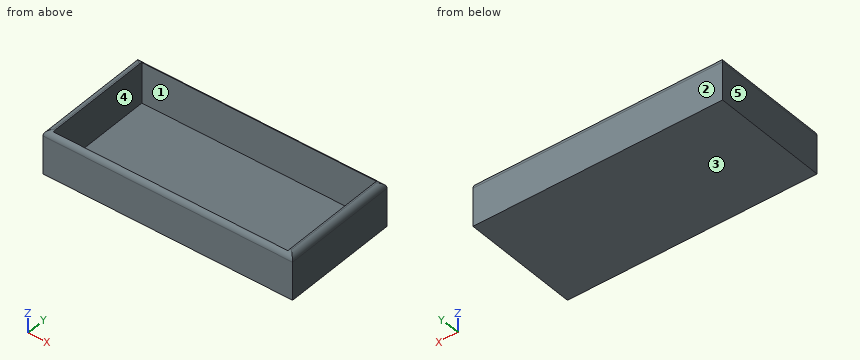
```python
from build123d import *

# Parameters (mm, degrees)
F0_W        = 170
F0_H        = 80
F1_DEPTH    = 30
F2_W        = 160
F2_H        = 75
F3_DEPTH    = 28
F4_T1_DEPTH = 190
F4_T3_DEPTH = 100


# Not quite as in the source:
# - a fillet or chamfer that OpenCascade refuses, or shapes differently, is made with other operations: its cross-section is extruded or revolved along the edge and cut away or added


with BuildPart() as f1:
    # F0 (on Top) → F1 (new body)
    with BuildSketch(Plane.XY):
        Rectangle(F0_W, F0_H)
    extrude(amount=F1_DEPTH)

    # F2 (on face) → F3 (cut)
    with BuildSketch(Plane.XY.offset(30)):
        Rectangle(F2_W, F2_H)
    extrude(amount=-F3_DEPTH, mode=Mode.SUBTRACT)

    # F4: fillet of radius 4 on 4 edges, made by hand

    # F4_s2 → F4_t1 (cut)
    with BuildSketch(Plane.YZ.offset(-95)):
        with BuildLine():
            ThreePointArc((-40, 26), (-38.8284271247, 28.8284271247), (-36, 30))
            Line((-36, 30), (-40, 30))
            Line((-40, 30), (-40, 26))
        make_face()
        with BuildLine():
            ThreePointArc((40, 26), (38.8284271247, 28.8284271247), (36, 30))
            Line((36, 30), (40, 30))
            Line((40, 30), (40, 26))
        make_face()
    extrude(amount=F4_T1_DEPTH, mode=Mode.SUBTRACT)

    # F4_s4 → F4_t3 (cut)
    with BuildSketch(Plane.XZ.offset(-50)):
        with BuildLine():
            ThreePointArc((-85, 26), (-83.8284271247, 28.8284271247), (-81, 30))
            Line((-81, 30), (-85, 30))
            Line((-85, 30), (-85, 26))
        make_face()
        with BuildLine():
            ThreePointArc((81, 30), (83.8284271247, 28.8284271247), (85, 26))
            Line((85, 26), (85, 30))
            Line((85, 30), (81, 30))
        make_face()
    extrude(amount=F4_T3_DEPTH, mode=Mode.SUBTRACT)


solid = f1.part
```
Source: CAD feature listing. Evaluate the final solid. Frame: model axes, mm. Face numbers are marked on the shaded views. A direction names the side the tool comes from. Round coordinates to 2 decimals unless told otherwise and drop trailing zeros. Write each loop counter-clockwise with the first axis right and the second up, starting at its lowest first coordinate (ties: lowest second). Pieces come first, ordered by that corner, then holes. Notation, with made-up numbers: M 26,88.5 L 32,88.5 A34 ccw 32,126.5 Z; hole C 33.25,42.5 d4. An arc over 180 degrees is marked long. Use CSV: the item, a comma, the result in double quotes. Start each with the question number.
Q1. Access query for the marked faces 1 and 2. Directions: +Z, -Z, +X, -X, +Y, -Y. A direction counts if a zero-diameter tool reaches every point of the face in a straight line with its end or side. Return the directions, or none.
Q2. First-contact query: P1, Ø4, axis at x = 64, y = -18.5, coming from the +Z side. Flat tip, straight axial feed; report the tip coordinate or a pass-through.
Q3. Cut plane B-B on x = -6.5. Output: boundary loops of the cut face in (y, z).
Q4. Line query: line 1 (Y direction, x = -6, z = 22.5); line 2 (X direction, y = -1.5, z = 12.5); line 3 (Z direction, x = -46, y = 3.5). Output: solid intervals per line, ascending. Write a range as from..to.
Q5. Cut plane A-A on z = 21. Output: boundary loops of the cut face in (x, y), plus the area to 3 significant figures.
Q6. Cut plane C-C on y = 17. Output: boundary loops of the cut face in (x, z).
Q7. Pull-direction query (X, two-part tool) for the marked faces 3, 4 and 5; classes: +X half, -X half, draft (parallel to the pull), parting line (faces both ways), or undercut.
Results found:
1,face 1,"+Z"
1,face 2,"+Z, -Z, +X, -X, +Y"
2,P1,"z = 2"
3,outline,"M -40,0 L 40,0 L 40,26 A4 ccw 37.5,29.71 L 37.5,2 L -37.5,2 L -37.5,29.71 A4 ccw -40,26 Z"
4,line 1,"-40..-37.5, 37.5..40"
4,line 2,"-85..-80, 80..85"
4,line 3,"0..2"
5,outline,"M -85,-40 L 85,-40 L 85,40 L -85,40 Z; hole M -80,-37.5 L 80,-37.5 L 80,37.5 L -80,37.5 Z"
5,area,"1,600 mm^2"
6,outline,"M -85,0 L 85,0 L 85,26 A4 ccw 81,30 L 80,30 L 80,2 L -80,2 L -80,30 L -81,30 A4 ccw -85,26 Z"
7,face 3,"draft"
7,face 4,"undercut"
7,face 5,"-X half"
